Part model, mm, in its own coordinate system. A direction names the side the tool comes from. Give positions to 0.01 mm unless a question says otherwise; leave off trailing zeros. Write each loop counter-clockwise with the first axis right and the second up, starting at its lowest first coordinate (ties: lowest second). Pieces come first, ordered by that corner, then holes.
Autodesk Inventor part; units mm, degrees
ref_plane "Work Plane1" through (0, -19, -18) normal (0, -1, 0) x (1, 0, 0)
ref_plane "YZ Plane" through (0, 0, 0) normal (1, 0, 0) x (0, 1, 0)
ref_plane "XZ Plane" through (0, 0, 0) normal (0, 1, 0) x (-1, 0, 0)
sketch "Sketch1" plane through (0, 0, 0) normal (0, 0, 1) x (1, 0, 0)
  circle A0 centre (0, 0) radius 3
  line L0 (0, 3) -> (0, 3)
  line L1 (-1.6583, 2.5) -> (1.6583, 2.5)
  line L2 (1.6583, 2.5) -> (1.6583, 4.0802)
  line L3 (-1.6583, 4.0802) -> (-1.6583, 2.5)
  point P0 (0, 2.5)
  dimension "d0" = 6
  dimension "d3" = 2.5
  dimension "d4" = 0
  dimension "d5" = 0.5
extrude "Extrusion1" add sketch "Sketch1" against normal blind 13 contours A0 L1 picked at (0.1141, 0.6732)
sketch "Sketch2" plane through (0, 0, -13) normal (0, 0, -1) x (-1, 0, 0)
  circle A0 centre (0, 0) radius 10
  dimension "d8" = 20
extrude "Extrusion2" add sketch "Sketch2" along normal blind 5
sketch "Sketch3" plane through (0, 0, -18) normal (0, 0, -1) x (-1, 0, 0)
  circle A0 centre (0, 0) radius 19
  dimension "d11" = 38
extrude "Extrusion3" add sketch "Sketch3" along normal blind 35
sketch "Sketch4" plane through (0, 0, -18) normal (0, 0, 1) x (1, 0, 0)
  arc A0 (-1.6583, 2.5) -> (1.6583, 2.5) centre (0, 0) ccw
  circle A1 centre (0, 0) radius 14
  circle A2 centre (0, 14) radius 1.25
  circle A3 centre (-12.1244, -7) radius 1.25
  circle A4 centre (12.1244, -7) radius 1.25
  circle A5 centre (0, 0) radius 15
  circle A6 centre (7.5, 12.9904) radius 1.25
  circle A7 centre (-15, 0) radius 1.25
  circle A8 centre (7.5, -12.9904) radius 1.25
  dimension "d14" = 28
  dimension "d20" = 30
  dimension "d15" = 2.5
  dimension "d18" = 360
  dimension "d21" = 2.5
  dimension "d22" = 30
  dimension "d25" = 360
extrude "Extrusion4" cut sketch "Sketch4" against normal blind 1 contours A6 A1 | A1 A6 A5 | A4 A5 A1 | A1 A4 | A5 A6 | A4 A5 | A2 A1 | A1 A2 A5 | A8 A5 A1 | A1 A8 | A5 A2 | A8 A5 | A7 A1 | A1 A7 A5 | A3 A5 A1 | A1 A3 | A5 A7 | A3 A5
sketch "Sketch5" plane through (0, 0, -18) normal (0, 0, 1) x (1, 0, 0)
  circle A0 centre (0, 0) radius 19
  point P0 (0, -19)
ref_plane "Work Plane1" through (0, -19, -18) normal (0, -1, 0) x (1, 0, 0)
sketch "Sketch6" plane through (0, -19, -18) normal (0, -1, 0) x (1, 0, 0)
  circle A0 centre (0, -26.2836) radius 5
  point P0 (0, 18)
  dimension "d29" = 10
extrude "Extrusion5" add sketch "Sketch6" along normal blind 5 and the other way blind 0.7
sketch "Sketch7" plane through (0, 0, -13) normal (0, 0, 1) x (1, 0, 0)
  circle A0 centre (0, 0) radius 3
extrude "Extrusion6" add sketch "Sketch7" along normal blind 3
equation "\"BendRadius\" = Thickness"
equation "\"BendReliefWidth\" = Thickness"
equation "\"BendReliefDepth\" = 0.5 * Thickness"
equation "\"CornerReliefSize\" = 4 * Thickness"
equation "\"MinimumRemnant\" = 2 * Thickness"
equation "\"TransitionRadius\" = BendRadius"
equation "\"JacobiRadiusSize\" = BendRadius"
equation "\"GapSize\" = Thickness"
properties part number "Optical Encoder"
1) Saw through at B-B (y = -7). Write the cut outline in (x, z).
Check result:
outline: (-17.66, -53) - (17.66, -53) - (17.66, -18) - (13.37, -18) - (13.37, -19) - (10.87, -19) - (10.87, -18) - (7.14, -18) - (7.14, -13) - (-7.14, -13) - (-7.14, -18) - (-10.87, -18) - (-10.87, -19) - (-13.37, -19) - (-13.37, -18) - (-17.66, -18) - close
2) Mould opens along Y. For faces 1 (the flat face through (0, 2.5, -5)), 2 (the flat face through (-12, -7, -19)), 3 (the cylindrical face through (4.119, 18.548, -35.255)), 4 (the flat face through (-2.1, 2.4, -13)) say: +Y half, -Y half, draft (parallel to the pull), parting line (faces both ways), or undercut.
Check result:
face 1: +Y half
face 2: undercut
face 3: parting line
face 4: draft
3) Saw through at D-D (x = -12). Write the cut outline in (y, z).
Check result:
outline: (-14.73, -53) - (14.73, -53) - (14.73, -18) - (-5.76, -18) - (-5.76, -19) - (-8.24, -19) - (-8.24, -18) - (-14.73, -18) - close
4) 3-axis set-ups, long thin cutter, end or side, ignore diameter. For faces 5 (the flat face through (0, 0, 0)), 6 (the cylindrical face through (6.508, -13.751, -18.493)): which of +Z, -Z, +X, -X, +Y, -Y reach the whole face in a straight line?
Check result:
face 5: +Z, +X, -X, +Y, -Y
face 6: +Z
5) Drill centre lines: L1, parallel to Y at x = 0, z = -18.45; L2, parallel to Z at x = -1, y = 10; L3, parallel to Z at x = 4, y = -1. Where is each one in solid material? Low to high.
Check result:
L1: y = -19 to 12.75, 15.25 to 19
L2: z = -53 to -18
L3: z = -53 to -13
6) Saw through at C-C (z = -20.5). Write the cut outline in (x, y), and give its area (3 significant figures).
Check result:
outline: circle Ø38 at (0, 0)
area: 1,130 mm2
7) Saw through at A-A (x = 0). Write the cut outline in (y, z).
Check result:
outline: (-24, -49.28) - (-19, -49.28) - (-19, -53) - (19, -53) - (19, -18) - (15.25, -18) - (15.25, -19) - (12.75, -19) - (12.75, -18) - (10, -18) - (10, -13) - (3, -13) - (3, -10) - (2.5, -10) - (2.5, 0) - (-3, 0) - (-3, -13) - (-10, -13) - (-10, -18) - (-19, -18) - (-19, -39.28) - (-24, -39.28) - close
8) Flat gauge pins, fed straight in: P1, Ø3, axis at x = 7, y = -12.5, coming from the +Z side; P2, Ø1.5, axis at x = 12.12, y = -7, coming from the +Z side; P3, Ø5, axis at y = -15, z = -38, coming from the +X side. Where does each tip first touch, or does it go through?
Check result:
P1: stops at z = -18
P2: stops at z = -19
P3: stops at x = 14.31
